Design review of the part built by this model. Coordinates are the model's own, in mm. Face numbers are marked on the shaded views. A direction names the side the tool comes from. Coordinates: 2 decimals unless noted, no trailing zeros. Order: outer loops, then holes, each group sorted by start corner. A loop starts at its lowest first (then second) coordinate and runs counter-clockwise, first axis right, second up. Notation, with made-up numbers: (-12.5, 61.25) -> (10.5, 61.25) arc R30 cw to (10.5, 83.25) -> close; hole circle Ø2 at (-24, 17.25). An arc over 180 degrees is marked (long way). Use a Markdown table: item, result. Add a question column.
Q1. Add section C-C (x = 17). State the section outline as (y, z) points, then the cut area to 3 significant figures.
Q2. Insertion check: pin 1 (8 mm diameter, centred on x = 2, y = 21, fed in from +Z); pin 2 (4 mm diameter, centred on y = -1.5, z = 28.5, fed in from +X); pin 3 (0.5 mm diameter, centred on x = 31, y = 10.5, fed in from +Z). Each pin has a flat end and moves straight along its axis. Give the tip position at first contact, or say it passes through.
Q3. Add section A-A (y = 0). State the section outline as (x, z) points, then the cut area to 3 significant figures.
Q4. Add section D-D (z = 26). State the section outline as (x, y) points.
Q5. Wall thickness on probe 1 along X at (y, z) = (23, 18); probe 2 along Z at (x, y) = (-30.9, 0); probe 3 along X at (y, z) = (34, 42.5): over which ranges is each line inside the solid? List them lowest first.
Q6. Add section B-B (z = 2). State the section outline as (x, y) points, then the cut area to 3 significant figures.
Q7. Machinability: for the marked faces 4 and 5, which of the approach directions +Z, -Z, +X, -X, +Y, -Y give a long, thin tool a straight path to every point of the face, cutting with its end or side? Answer none if there is none.
Q8. The part is to be moulded in two halves that separate along X. For the marked faces 1, 2 and 3, say which applies: pulls with the +X half, pulls with the -X half, needs draft (parallel to the pull), parting line crosses it, or undercut.
from build123d import *

# Parameters (mm, degrees)
SCHIZZO1_W                   = 64
SCHIZZO1_H                   = 98
ESTRUSIONE_ESTRUSIONE1_DEPTH = 2
SCHIZZO4_W                   = 2
SCHIZZO4_H                   = 98
ESTRUSIONE_ESTRUSIONE2_DEPTH = 45
SCHIZZO5_W                   = 2
SCHIZZO5_H                   = 98
ESTRUSIONE_ESTRUSIONE3_DEPTH = 20
RACCORDO1_R                  = 0.5
SCHIZZO6_R                   = 4
TAGLIO_ESTRUSIONE1_DEPTH     = 10


with BuildPart() as part:
    # Schizzo1 → Estrusione-Estrusione1 (new body)
    with BuildSketch(Plane.XY):
        Rectangle(SCHIZZO1_W, SCHIZZO1_H)
    extrude(amount=-ESTRUSIONE_ESTRUSIONE1_DEPTH)

    # Schizzo4 → Estrusione-Estrusione2 (add)
    with BuildSketch(Plane.XY):
        with Locations((-31, 0)):
            Rectangle(SCHIZZO4_W, SCHIZZO4_H)
    extrude(amount=ESTRUSIONE_ESTRUSIONE2_DEPTH)

    # Schizzo5 → Estrusione-Estrusione3 (add)
    with BuildSketch(Plane.XY):
        with Locations((31, 0)):
            Rectangle(SCHIZZO5_W, SCHIZZO5_H)
    extrude(amount=ESTRUSIONE_ESTRUSIONE3_DEPTH)

    # Raccordo1
    raccordo1_edges = [part.edges().sort_by_distance(p)[0] for p in [
        (-30, 0, 0),
        (-32, 0, 45),
        (-30, 0, 45),
        (30, 0, 0),
        (32, 0, 20),
        (30, 0, 20),
    ]]
    fillet(raccordo1_edges, radius=RACCORDO1_R)

    # Schizzo6 → Taglio-Estrusione1 (cut)
    with BuildSketch(Plane.ZY.offset(32)):
        with Locations(Location((13.5, 0, 0), (0, 0, 270))):
            Circle(SCHIZZO6_R)
    extrude(amount=-TAGLIO_ESTRUSIONE1_DEPTH, mode=Mode.SUBTRACT)


solid = part.part
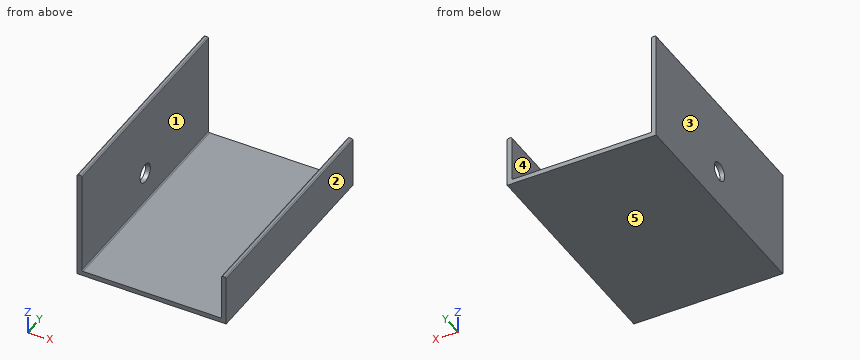
Established:
| question | item | result |
|---|---|---|
| 1 | outline | (-49, -2) -> (49, -2) -> (49, 0) -> (-49, 0) -> close |
| 1 | area | 196 mm^2 |
| 2 | pin 1 | z = 0 |
| 2 | pin 2 | x = -30 |
| 2 | pin 3 | z = 20 |
| 3 | outline | (-32, -2) -> (32, -2) -> (32, 19.5) arc R0.5 ccw to (31.5, 20) -> (30.5, 20) arc R0.5 ccw to (30, 19.5) -> (30, 0.5) arc R0.5 cw to (29.5, 0) -> (-29.5, 0) arc R0.5 cw to (-30, 0.5) -> (-30, 9.5) -> (-32, 9.5) -> close; (-32, 17.5) -> (-30, 17.5) -> (-30, 44.5) arc R0.5 ccw to (-30.5, 45) -> (-31.5, 45) arc R0.5 ccw to (-32, 44.5) -> close |
| 3 | area | 242 mm^2 |
| 4 | outline | (-32, -49) -> (-30, -49) -> (-30, 49) -> (-32, 49) -> close |
| 5 | probe 1 | -32 to -30, 30 to 32 |
| 5 | probe 2 | -2 to 9.5, 17.5 to 45 |
| 5 | probe 3 | -32 to -30 |
| 6 | outline | (-32, -49) -> (-30, -49) -> (-30, 49) -> (-32, 49) -> close; (30, -49) -> (32, -49) -> (32, 49) -> (30, 49) -> close |
| 6 | area | 392 mm^2 |
| 7 | face 4 | +Z, +Y, -Y |
| 7 | face 5 | -Z, +X, -X, +Y, -Y |
| 8 | face 1 | undercut |
| 8 | face 2 | pulls with the +X half |
| 8 | face 3 | pulls with the -X half |
